Verification items for the finished model (mm, model axes). A direction names the side the tool comes from. Round coordinates to 2 decimals unless told otherwise and drop trailing zeros. Write each loop counter-clockwise with the first axis right and the second up, starting at its lowest first coordinate (ties: lowest second). Pieces come first, ordered by that corner, then holes. Notation, with made-up numbers: (45.5, -15.75) -> (85.5, -15.75) arc R19 cw to (85.5, -2.75) -> close; hole circle Ø7 at (84, 81.5). An arc over 180 degrees is marked (long way). Answer as a JSON object with one key per item and string values. Group by question number.
(1) Scan lines: L1, parallel to Y at x = 27.5, z = 20.5 (3 decimals); L2, parallel to Z at x = 12, y = -13; L3, parallel to X at y = -16.5, z = 26. Record each from-to range of solid material in increasing order. Write a range as from..to.
(2) Set-up check for faces 5 (the face through (-35.55, -19.86, 28.59)), 6 (the face through (29, -26.575, 29)), 7 (the face through (-11.05, -20, 26)): record each of +Z, -Z, +X, -X, +Y, -Y from which the full face is reachable in a straight line by a thin tool's end or side.
(3) Sectioned sample at A-A on z = 21.5. Record the cut outline in (x, y) (3 decimals).
(4) Gauge pin test, flat ends, axial feed: pin 1 Ø10.5 at (y, z) = (-23, 31) entering from +X; pin 2 Ø9 at (x, z) = (-23, 28.5) entering from +Y (3 decimals); pin 3 Ø9 at (x, z) = (31, 25.5) entering from -Y (3 decimals). Record the tip position at first contact, or that the pin passes through.
(5) Draft check along Y on faces 1 (the face through (4, -20, 12.731)), 2 (the face through (4, -40, 14)), 3 (the face through (4, -13.65, 16)), 4 (the face through (-23, -20, 38.731)). Enter one of: released by +Y, released by -Y, zero draft, split by the parting line, or undercut.
(6) Sectioned sample at D-D on y = -15. Record the cut outline in (x, z).
(7) Sectioned sample at C-C on y = -20. Record the cut outline in (x, z).
(8) Sectioned sample at B-B on x = -26.5. Record the cut outline in (y, z) (3 decimals).
```python
from build123d import *

# Parameters (mm, degrees)
F0_W     = 90
F0_H     = 40
F1_DEPTH = 10
F2_W     = 31
F2_H     = 12.7
F3_DEPTH = 6
F5_DEPTH = 20
F6_ANGLE = 270


with BuildPart() as f1:
    # F0 (on Front) → F1 (new body)
    with BuildSketch(Plane.XZ):
        with Locations((4.450109, -11.269131)):
            Rectangle(F0_W, F0_H)
    extrude(amount=F1_DEPTH)

    # F2 (on face) → F3 (cut)
    with BuildSketch(Plane.XZ.offset(10)):
        with Locations((4.450109, -11.269131)):
            Rectangle(F2_W, F2_H)
    extrude(amount=-F3_DEPTH, mode=Mode.SUBTRACT)

    # F4 (on face) → F5 (join)
    with BuildSketch(Plane.XZ.offset(10)):
        with BuildLine():
            ThreePointArc((37.875109, -17.844131), (44.450109, -11.269131), (37.875109, -4.694131))
            Line((37.875109, -4.694131), (19.950109, -4.694131))
            Line((19.950109, -4.694131), (19.950109, -17.844131))
            Line((19.950109, -17.844131), (37.875109, -17.844131))
        make_face()
        with BuildLine():
            Line((-28.974891, -17.844131), (-11.049891, -17.844131))
            Line((-11.049891, -17.844131), (-11.049891, -4.694131))
            Line((-11.049891, -4.694131), (-28.974891, -4.694131))
            ThreePointArc((-28.974891, -4.694131), (-35.549891, -11.269131), (-28.974891, -17.844131))
        make_face()
    extrude(amount=F5_DEPTH)


with BuildPart() as f1_1:
    # F6: moved
    add(f1.part.rotate(Axis((4.450109, 0, 8.730869), (1, 0, 0)), F6_ANGLE))


solid = f1_1.part
```
Computed values:
{
 "1": {"L1": "-26.575..-13.425", "L2": "8.73..18.73", "L3": "-34.54..-11.05, 19.95..43.44"},
 "2": {"face 5": "+Z, -X", "face 6": "+Z, +X, -X, -Y", "face 7": "+Z"},
 "3": {"outline": "(-28.975, -26.575) -> (-11.05, -26.575) -> (-11.05, -13.425) -> (-28.975, -13.425) arc R6.575 ccw to start; (19.95, -26.575) -> (37.875, -26.575) arc R6.575 ccw to (37.875, -13.425) -> (19.95, -13.425) -> close"},
 "4": {"pin 1": "x = 44.45", "pin 2": "y = -13.425", "pin 3": "y = -26.575"},
 "5": {"face 1": "undercut", "face 2": "released by -Y", "face 3": "undercut", "face 4": "zero draft"},
 "6": {"outline": "(-40.55, 8.73) -> (49.45, 8.73) -> (49.45, 18.73) -> (42.14, 18.73) -> (42.14, 38.73) -> (19.95, 38.73) -> (19.95, 12.73) -> (-11.05, 12.73) -> (-11.05, 38.73) -> (-33.24, 38.73) -> (-33.24, 18.73) -> (-40.55, 18.73) -> close"},
 "7": {"outline": "(-40.55, 8.73) -> (49.45, 8.73) -> (49.45, 18.73) -> (44.45, 18.73) -> (44.45, 38.73) -> (19.95, 38.73) -> (19.95, 12.73) -> (-11.05, 12.73) -> (-11.05, 38.73) -> (-35.55, 38.73) -> (-35.55, 18.73) -> (-40.55, 18.73) -> close"},
 "8": {"outline": "(-40, 8.731) -> (0, 8.731) -> (0, 18.731) -> (-13.425, 18.731) -> (-13.425, 38.731) -> (-26.575, 38.731) -> (-26.575, 18.731) -> (-40, 18.731) -> close"}
}
